Check sheet for the modelled part. Datum: model origin and axes. Units: mm. A direction names the side the tool comes from. Round coordinates to 2 decimals unless told otherwise and drop trailing zeros. Write each loop counter-clockwise with the first axis right and the second up, starting at its lowest first coordinate (ties: lowest second). Pieces come first, ordered by that corner, then holes. Notation, with made-up numbers: M 38.25,76.5 L 87.25,76.5 A25 cw 87.25,101.5 Z; hole C -15.75,35 d6. An arc over 180 degrees is marked long. One line per item, written item: value.
from build123d import *

# Parameters (mm, degrees)
PAD_DEPTH       = 11
SKETCH002_R     = 1.5
PAD001_DEPTH    = 2.5
POCKET_DEPTH    = 5
SKETCH004_W     = 2
SKETCH004_H     = 0.5
SKETCH004_W_2   = 0.5
SKETCH004_H_2   = 3.85
PAD002_DEPTH    = 2
SKETCH005_W     = 14
SKETCH005_H     = 7
SKETCH005_W_2   = 16
SKETCH005_H_2   = 3
POCKET001_DEPTH = 4


with BuildPart() as part:
    # Sketch001 → Pad (new body, symmetric)
    with BuildSketch(Plane.YZ):
        with BuildLine():
            Line((-12, 0), (12, 0))
            Line((12, 0), (12, 5.35))
            ThreePointArc((12, 5.35), (11.707107, 6.057107), (11, 6.35))
            Line((11, 6.35), (-5.65, 6.35))
            Line((-5.65, 6.35), (-12, 0))
        make_face()
    extrude(amount=PAD_DEPTH, both=True)

    # Sketch002 (on Face7 of Pad) → Pad001 (join)
    with BuildSketch(Plane.YZ.offset(11)):
        with Locations((9.5, 3.85)):
            Circle(SKETCH002_R)
    pad001 = extrude(amount=PAD001_DEPTH)

    # Sketch003 (on Face3 of Pad001) → Pocket (cut)
    with BuildSketch(Plane.ZX.offset(12)):
        Polygon((4.35, 13.5), (5.35, 13.5), (5.35, 12.5), align=None)
    pocket = extrude(amount=-POCKET_DEPTH, mode=Mode.SUBTRACT)

    # Sketch004 (on Face5 of Pocket) → Pad002 (join)
    with BuildSketch(Plane.YZ.offset(11)):
        with Locations((11, 3.85)):
            Rectangle(SKETCH004_W, SKETCH004_H)
        with Locations((9.5, 1.925)):
            Rectangle(SKETCH004_W_2, SKETCH004_H_2)
    pad002 = extrude(amount=PAD002_DEPTH)

    # Mirrored: Pad002, Pocket, Pad001 across YZ
    add(pad002.mirror(Plane.YZ))
    add(pocket.mirror(Plane.YZ), mode=Mode.SUBTRACT)
    add(pad001.mirror(Plane.YZ))

    # Sketch005 (on Face10 of Mirrored) → Pocket001 (cut)
    with BuildSketch(Plane(origin=(0, 0, 6.35), x_dir=(0, -1, 0), z_dir=(0, 0, 1))):
        with Locations((-3, 0)):
            Rectangle(SKETCH005_W, SKETCH005_H)
        with Locations((-8, 7.5)):
            Rectangle(SKETCH005_W_2, SKETCH005_H_2)
        with Locations((-8, -7.5)):
            Rectangle(SKETCH005_W_2, SKETCH005_H_2)
    extrude(amount=-POCKET001_DEPTH, mode=Mode.SUBTRACT)


solid = part.part
Q1. Depth check by flat-ended pin: P1, Ø0.9, axis at x = 7, z = 4, coming from the +Y side; P2, Ø1.6, axis at x = 12.5, z = 0.5, coming from the -Y side; P3, Ø0.8, axis at x = -12, y = 11.5, coming from the +Z side. Enter the tip coordinate at first touch or a pass-through.
Completed:
P1: y = 0
P2: y = 9.25
P3: z = 4.1
Q2. Sectioned sample at B-B on x = -4.75. Enter the section's corners in (y, z).
Completed:
outline: M -12,0 L 12,0 L 12,5.35 A1 ccw 11,6.35 L -5.65,6.35 Z
Q3. Draft check along X on faces 5 (the flat face through (7, 0, 4)), 6 (the flat face through (-12, 9.25, 1)), 7 (the flat face through (-11, 11, 1)), 8 (the flat face through (-8, 0, 4)). Enter one of: pulls with the +X half, pulls with the -X half, needs draft (parallel to the pull), parting line crosses it, or undercut.
Completed:
face 5: undercut
face 6: needs draft
face 7: pulls with the -X half
face 8: undercut
Q4. Scan lines: line 1 (X direction, y = 0.5, z = 4.5); line 2 (X direction, y = 9.25, z = 4); line 3 (X direction, y = 8.75, z = 1). Record each from-to range of solid material in increasing order. Write a range as [from, to].
Completed:
line 1: [-11, -9], [-6, -3.5], [3.5, 6], [9, 11]
line 2: [-13.5, -9], [-6, -3.5], [3.5, 6], [9, 13.5]
line 3: [-11, 11]
Q5. Sectioned sample at C-C on z = 0.5. Enter the section's corners in (x, y).
Completed:
outline: M -13,9.25 L -11,9.25 L -11,-11.5 L 11,-11.5 L 11,9.25 L 13,9.25 L 13,9.75 L 11,9.75 L 11,12 L -11,12 L -11,9.75 L -13,9.75 Z
Q6. Sectioned sample at A-A on y = 6.25. Enter the section's corners in (x, z).
Completed:
outline: M -11,0 L 11,0 L 11,6.35 L 9,6.35 L 9,2.35 L 6,2.35 L 6,6.35 L 3.5,6.35 L 3.5,2.35 L -3.5,2.35 L -3.5,6.35 L -6,6.35 L -6,2.35 L -9,2.35 L -9,6.35 L -11,6.35 Z
Q7. Sectioned sample at D-D on z = 3. Enter the section's corners in (x, y).
Completed:
outline: M -13.5,8.26 L -11,8.26 L -11,-9 L 11,-9 L 11,8.26 L 13.5,8.26 L 13.5,10.74 L 11,10.74 L 11,12 L 9,12 L 9,0 L 6,0 L 6,12 L -6,12 L -6,0 L -9,0 L -9,12 L -11,12 L -11,10.74 L -13.5,10.74 Z; hole M -3.5,-4 L 3.5,-4 L 3.5,10 L -3.5,10 Z
Q8. Access from +Z, -Z, +X, -X, +Y, -Y to the whole of each face (thin tool, end or side, straight path). Record for faces 1 (the cylindrical face through (-12.23, 8.31, 2.94)), 2 (the flat face through (-9, 6, 4)), 3 (the flat face through (11, 11, 1)), 4 (the cylindrical face through (12.23, 10.19, 2.52)).
Completed:
face 1: -X
face 2: +Z, +Y
face 3: -Z, +X, +Y
face 4: +X
